Autodesk Inventor part; units mm, degrees
ref_plane "YZ Plane" through (0, 0, 0) normal (1, 0, 0) x (0, 1, 0)
ref_plane "XZ Plane" through (0, 0, 0) normal (0, 1, 0) x (-1, 0, 0)
ref_plane "XY Plane" through (0, 0, 0) normal (0, 0, 1) x (1, 0, 0)
sketch "Náčrt1" plane through (0, 0, 0) normal (0, 0, 1) x (1, 0, 0)
  line L0 (0, 0) -> (0, 32)
  line L1 (0, 0) -> (35, 0)
  circle A0 centre (10.5, 5) radius 1.1
  circle A1 centre (10.5, 17.5) radius 1.1
  line L2 (0, 12) -> (7, 12)
  line L3 (7, 12) -> (7, 24)
  line L4 (7, 24) -> (35, 24)
  line L5 (35, 24) -> (35, 0)
  line L6 (0, 0) -> (-35, 0)
  circle A2 centre (-10.5, 5) radius 1.1
  circle A3 centre (-10.5, 17.5) radius 1.1
  line L7 (0, 12) -> (-7, 12)
  line L8 (-7, 12) -> (-7, 24)
  line L9 (-7, 24) -> (-35, 24)
  line L10 (-35, 24) -> (-35, 0)
  dimension "d0" = 32
  dimension "d1" = 35
  dimension "d2" = 2.2
  dimension "d3" = 5
  dimension "d4" = 10.5
  dimension "d5" = 2.2
  dimension "d6" = 12.5
  dimension "d7" = 12
  dimension "d8" = 7
  dimension "d9" = 12
extrude "Vysunutí1" add sketch "Náčrt1" along normal blind 2.5
sketch "Náčrt2" plane through (0, 0, 2.5) normal (0, 0, 1) x (1, 0, 0)
  line L0 (7, 12) -> (-7, 12)
  line L1 (0, 12) -> (-35, 12)
  line L2 (-35, 24) -> (-35, 0)
  circle A0 centre (-32, 12) radius 2.55
  circle A1 centre (-26, 12) radius 2.55
  circle A2 centre (-20, 12) radius 2.55
  line L3 (-7, 12) -> (-7, 24)
  line L4 (0, 0) -> (0, 12)
  circle A3 centre (32, 12) radius 2.55
  circle A4 centre (26, 12) radius 2.55
  circle A5 centre (20, 12) radius 2.55
  dimension "d12" = 5.1
  dimension "d17" = 13
  dimension "d18" = 5.1
  dimension "d19" = 5.1
  dimension "d20" = 6
  dimension "d21" = 6
extrude "Vysunutí2" cut sketch "Náčrt2" against normal through all
properties part number "kamera2"
Could you check a few things on this model? Use its own coordinates, in mm. A direction names the side the tool comes from. Give positions to 0.01 mm unless a question says otherwise; leave off trailing zeros. Loops run counter-clockwise (first coordinate to the right, second up) from the corner with the lowest first, then second, coordinate; pieces in that order, holes last. Notation, with made-up numbers: (19.5, 55) -> (42.5, 55) arc R19 ccw to (42.5, 87) -> close; hole circle Ø1 at (63, 73). An arc over 180 degrees is marked (long way). Return JSON: item names as keys, results as strings.
Item 1: If we section it at C-C on y = 5: List the corners of the cut face in (x, z) for me, plus the area to 3 significant figures.
Geometry results:
{"outline": "(-35, 0) -> (-11.6, 0) -> (-11.6, 2.5) -> (-35, 2.5) -> close; (-9.4, 0) -> (9.4, 0) -> (9.4, 2.5) -> (-9.4, 2.5) -> close; (11.6, 0) -> (35, 0) -> (35, 2.5) -> (11.6, 2.5) -> close", "area": "164 mm²"}
Item 2: If we section it at A-A on z = 0.4: Count the separate pieces of the cut face and the enclosed holes in it, plus the area to 3 significant figures.
Geometry results:
{"separate pieces": "1", "enclosed holes": "10", "area": "1,370 mm²"}
Item 3: Which directions (+Z, -Z, +X, -X, +Y, -Y) give clear straight access to the entire face, cutting with the end or side of a thin tool? Please do faces 4 (the cylindrical face through (11.55, 4.67, 1.23)), 5 (the flat face through (7, 18, 1)).
Geometry results:
{"face 4": "+Z, -Z", "face 5": "+Z, -Z, +Y"}
Item 4: If we section it at B-B on x = 20: List the corners of the cut face in (y, z) for me.
Geometry results:
{"outline": "(0, 0) -> (9.45, 0) -> (9.45, 2.5) -> (0, 2.5) -> close; (14.55, 0) -> (24, 0) -> (24, 2.5) -> (14.55, 2.5) -> close"}
Item 5: If we section it at D-D on y = 17.5: List the corners of the cut face in (x, z) for me, plus the area to 3 significant figures.
Geometry results:
{"outline": "(-35, 0) -> (-11.6, 0) -> (-11.6, 2.5) -> (-35, 2.5) -> close; (-9.4, 0) -> (-7, 0) -> (-7, 2.5) -> (-9.4, 2.5) -> close; (7, 0) -> (9.4, 0) -> (9.4, 2.5) -> (7, 2.5) -> close; (11.6, 0) -> (35, 0) -> (35, 2.5) -> (11.6, 2.5) -> close", "area": "129 mm²"}
Item 6: I need wall thicknesses on L1, parallel to Y at x = 10.5, z = 1.8; L2, parallel to Y at x = -26, z = 0.9; L3, parallel to X at y = 5.5, z = 0.95. Which ranges of each line are inside material? Lowest first, please. Write a range as from..to.
Geometry results:
{"L1": "y = 0..3.9, 6.1..16.4, 18.6..24", "L2": "y = 0..9.45, 14.55..24", "L3": "x = -35..-11.48, -9.52..9.52, 11.48..35"}
Item 7: I'm going to push flat-ended pins straight in: pin 1 (4 mm diameter, centred on x = 26, y = 12, fed in from +Z); pin 2 (0.8 mm diameter, centred on x = 1, z = 1.5, fed in from +Y). Where does each tip first touch, or does it pass through?
Geometry results:
{"pin 1": "passes through", "pin 2": "stops at y = 12"}
Item 8: We'd pull the mould along Y, two halves only. Please class faces 1 (the flat face through (0, 0, 1)), 2 (the flat face through (0, 10, 2.5)), 3 (the cylindrical face through (-28.024, 10.448, 1.268)): +Y half, -Y half, draft (parallel to the pull), parting line (faces both ways), or undercut.
Geometry results:
{"face 1": "-Y half", "face 2": "draft", "face 3": "undercut"}
